Autodesk Fusion 360 part; units mm, degrees
sketch "Sketch1" plane through (0, 0, 0) normal (0, 1, 0) x (1, 0, 0)
  circle A0 centre (0, 0) radius 22.5
  line L0 (-30.5533, 17.0732) -> (-13.0943, 48.3171)
  arc A1 (13.0943, 48.3171) -> (-13.0943, 48.3171) centre (0, 41) ccw
  line L1 (13.0943, 48.3171) -> (30.5533, 17.0732)
  arc A2 (-30.5533, 17.0732) -> (30.5533, 17.0732) centre (0, 0) ccw
  circle A3 centre (0, 41) radius 5
  point P0 (0, 29.35)
  dimension "d1" = 45
  dimension "d2" = 41
  dimension "d3" = 10
  dimension "d4" = 35
  dimension "d5" = 15
  dimension "d8" = 29.35
extrude "Extrude1" add sketch "Sketch1" along normal blind 2.5
hole "Hole1" at (0, 0, -29.35) direction (0, 1, 0) diameter 6.6 end through all
pattern_circular "C-Pattern1" count 12 over 360 about axis through (0, 1.75, 0) along (0, 1, 0) of "Hole1"
equation "d8 = ( 58.7 / 2 ) * 1 mm"
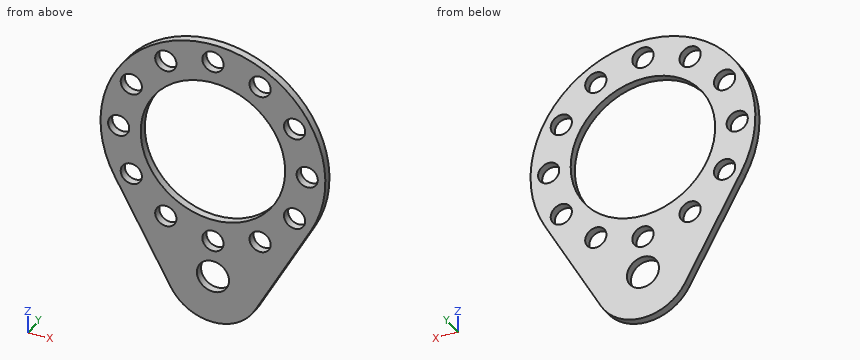
CAD build for the part. Positions are in the model's coordinates, mm. Coordinates: 2 decimals unless noted, no trailing zeros. Loops run counter-clockwise (first coordinate to the right, second up) from the corner with the lowest first, then second, coordinate; pieces in that order, holes last. Notation, with made-up numbers: (64.25, 42) - (70.25, 42) arc R28 cw to (70.25, 77) - close; hole circle Ø4 at (83.25, -9.5). An arc over 180 degrees is marked (long way). Return JSON: item names as keys, results as strings.
1. Band-saw the part on C-C (z = 14.5). Give the cut face in (x, y).
Result:
{"outline": "(-31.86, 0) - (-28.71, 0) - (-28.71, 2.5) - (-31.86, 2.5) - close; (-22.12, 0) - (-17.2, 0) - (-17.2, 2.5) - (-22.12, 2.5) - close; (17.2, 0) - (22.12, 0) - (22.12, 2.5) - (17.2, 2.5) - close; (28.71, 0) - (31.86, 0) - (31.86, 2.5) - (28.71, 2.5) - close"}
2. Band-saw the part on A-A (z = -39). Give the cut face in (x, y), and give its area (3 significant figures).
Result:
{"outline": "(-18.3, 0) - (-4.58, 0) - (-4.58, 2.5) - (-18.3, 2.5) - close; (4.58, 0) - (18.3, 0) - (18.3, 2.5) - (4.58, 2.5) - close", "area": "68.6 mm2"}
3. Drop a flat-ended pin along its axis: pin 1 (1.5 mm diameter, centred on x = -3, y = 1, fed in from -Z). Give the stop position or say it passes through.
Result:
{"pin 1": "stops at z = -55.83"}
4. Probe L1, parallel to Z at x = -13, y = 1.2; L2, parallel to X at y = 1.35, z = 16; L3, parallel to Z at x = 17, y = 0.2. List the from-to ranges inside material, lowest first. Write a range as from..to.
Result:
{"L1": "z = -48.48..-28.26, -22.57..-18.36, 18.36..22.57, 28.26..32.5", "L2": "x = -31.13..-28.44, -22.4..-15.82, 15.82..22.4, 28.44..31.13", "L3": "z = -41.33..-27.76, -23.08..-14.74, 14.74..23.08, 27.76..30.59"}
5. Band-saw the part on B-B (x = 0). Give the cut face in (y, z), and give its area (3 significant figures).
Result:
{"outline": "(0, -56) - (2.5, -56) - (2.5, -46) - (0, -46) - close; (0, -36) - (2.5, -36) - (2.5, -32.65) - (0, -32.65) - close; (0, -26.05) - (2.5, -26.05) - (2.5, -22.5) - (0, -22.5) - close; (0, 22.5) - (2.5, 22.5) - (2.5, 26.05) - (0, 26.05) - close; (0, 32.65) - (2.5, 32.65) - (2.5, 35) - (0, 35) - close", "area": "57.0 mm2"}
